Source: CAD feature listing. Evaluate the final solid. Frame: model axes, mm. Face numbers are marked on the shaded views. A direction names the side the tool comes from. Give positions to 0.01 mm unless a question says otherwise; leave off trailing zeros. Order: outer loops, then holes, each group sorted by start corner. A loop starts at its lowest first (then second) coordinate and runs counter-clockwise, first axis right, second up. Notation, with made-up numbers: M 78.5,-38.5 L 97.5,-38.5 A24 cw 97.5,-16.5 Z; hole C 33,-15 d11. An arc over 180 degrees is marked long. One line per question, with ' | ' between items. Start each with the question number.
from build123d import *

# Parameters (mm, degrees)
SKETCH_1_W               = 107
SKETCH_1_H               = 94
EXTRUDE_1_DEPTH          = 2
SKETCH_2_W               = 107
SKETCH_2_H               = 94
SKETCH_2_W_2             = 104
SKETCH_2_H_2             = 91
EXTRUDE_2_DEPTH          = 6.5
SKETCH_5_W               = 100
SKETCH_5_H               = 3.5
CUT_EXTRUDE_2_DEPTH      = 1.5
SKETCH_3_W               = 5
SKETCH_3_H               = 15
EXTRUDE_3_DEPTH          = 30
CUT_EXTRUDE_3_DEPTH      = 148.537283424
CUT_EXTRUDE_3_DEPTH_BACK = 30
SKETCH_6_W               = 3
SKETCH_6_H               = 9
SKETCH_7_W               = 10
SKETCH_7_H               = 15
EXTRUDE_4_DEPTH          = 2
SKETCH_8_R               = 1.5
CUT_EXTRUDE_4_DEPTH      = 2
CHAMFER_1_SIZE           = 0.5
EXTRUDE_5_DEPTH          = 3
EXTRUDE_6_DEPTH          = 3
EXTRUDE_7_DEPTH          = 3
MIRROR_2_COPY_1_DEPTH    = 3
EXTRUDE_8_DEPTH          = 15
EXTRUDE_9_DEPTH          = 15
EXTRUDE_10_DEPTH         = 9
EXTRUDE_11_DEPTH         = 9
EXTRUDE_12_DEPTH         = 3


with BuildPart() as part:
    # 草图1 → 凸台-拉伸1 (new body)
    with BuildSketch(Plane.XY):
        with Locations((53.5, -47)):
            Rectangle(SKETCH_1_W, SKETCH_1_H)
    extrude(amount=EXTRUDE_1_DEPTH)

    # 草图2 → 凸台-拉伸2 (add)
    with BuildSketch(Plane.XY.offset(2)):
        with Locations((53.5, -47)):
            Rectangle(SKETCH_2_W, SKETCH_2_H)
        with Locations((53.5, -47)):
            Rectangle(SKETCH_2_W_2, SKETCH_2_H_2, mode=Mode.SUBTRACT)
    extrude(amount=EXTRUDE_2_DEPTH)

    # 草图5 → 切除-拉伸2 (cut)
    with BuildSketch(Plane(origin=(0, -92.5, 0), x_dir=(1, 0, 0), z_dir=(0, 1, 0))):
        with Locations((53.5, -6.75)):
            Rectangle(SKETCH_5_W, SKETCH_5_H)
    extrude(amount=-CUT_EXTRUDE_2_DEPTH, mode=Mode.SUBTRACT)

    # 草图3 → 凸台-拉伸3 (add)
    with BuildSketch(Plane(origin=(0, 0, 0), x_dir=(-1, 0, 0), z_dir=(0, 0, -1))):
        with Locations((-2.5, -7.5)):
            Rectangle(SKETCH_3_W, SKETCH_3_H)
        with Locations((-104.5, -7.5)):
            Rectangle(SKETCH_3_W, SKETCH_3_H)
        with Locations((-2.5, -86.5)):
            Rectangle(SKETCH_3_W, SKETCH_3_H)
        with Locations((-104.5, -86.5)):
            Rectangle(SKETCH_3_W, SKETCH_3_H)
    extrude(amount=EXTRUDE_3_DEPTH)

    # 草图6 → 切除-拉伸3 (cut, two sides: drawn at the far end of the back side and taken through both)
    with BuildSketch(Plane(origin=(0, 0, -30), x_dir=(-1, 0, 0), z_dir=(0, 0, -1)).offset(-CUT_EXTRUDE_3_DEPTH_BACK)):
        with Locations((-103.5, -7.5)):
            Rectangle(SKETCH_6_W, SKETCH_6_H)
        with Locations((-103.5, -86.5)):
            Rectangle(SKETCH_6_W, SKETCH_6_H)
        with Locations((-3.5, -86.5)):
            Rectangle(SKETCH_6_W, SKETCH_6_H)
        with Locations((-3.5, -7.5)):
            Rectangle(SKETCH_6_W, SKETCH_6_H)
    extrude(amount=CUT_EXTRUDE_3_DEPTH + CUT_EXTRUDE_3_DEPTH_BACK, mode=Mode.SUBTRACT)

    # 草图7 → 凸台-拉伸4 (add)
    with BuildSketch(Plane(origin=(0, 0, -30), x_dir=(-1, 0, 0), z_dir=(0, 0, -1))):
        with Locations((5, -7.5)):
            Rectangle(SKETCH_7_W, SKETCH_7_H)
        with Locations((5, -86.5)):
            Rectangle(SKETCH_7_W, SKETCH_7_H)
        with Locations((-112, -7.5)):
            Rectangle(SKETCH_7_W, SKETCH_7_H)
        with Locations((-112, -86.5)):
            Rectangle(SKETCH_7_W, SKETCH_7_H)
    extrude(amount=-EXTRUDE_4_DEPTH)

    # 草图8 → 切除-拉伸4 (cut)
    with BuildSketch(Plane.XY.offset(-28)):
        with Locations((112.5, -7.5)):
            Circle(SKETCH_8_R)
        with Locations(Location((112.5, -86.5, 0), (0, 0, 180))):
            Circle(SKETCH_8_R)
        with Locations(Location((-5.5, -7.5, 0), (0, 0, 180))):
            Circle(SKETCH_8_R)
        with Locations((-5.5, -86.5)):
            Circle(SKETCH_8_R)
    extrude(amount=-CUT_EXTRUDE_4_DEPTH, mode=Mode.SUBTRACT)

    # 倒角1
    chamfer_1_edges = [part.edges().sort_by_distance(p)[0] for p in [
        (114, -86.5, -28),
        (-4, -7.5, -28),
        (-7, -86.5, -28),
        (111, -7.5, -28),
    ]]
    chamfer(chamfer_1_edges, length=CHAMFER_1_SIZE)

    # 草图9 → 凸台-拉伸5 (add)
    with BuildSketch(Plane.XZ.offset(94)):
        Polygon((87, 0), (102, -10), (102, 0), align=None)
        Polygon((5, 0), (20, 0), (5, -10), align=None)
    extrude_5 = extrude(amount=-EXTRUDE_5_DEPTH)

    # 草图10 → 凸台-拉伸6 (add)
    with BuildSketch(Plane(origin=(0, -79, 0), x_dir=(1, 0, 0), z_dir=(0, 1, 0))):
        Polygon((102, 10), (87, 0), (102, 0), align=None)
        Polygon((5, 0), (5, 10), (20, 0), align=None)
    extrude_6 = extrude(amount=-EXTRUDE_6_DEPTH)

    # 草图11 → 凸台-拉伸7 (add)
    with BuildSketch(Plane.ZY):
        Polygon((-20, -79), (0, -69), (0, -79), align=None)
    extrude_7 = extrude(amount=-EXTRUDE_7_DEPTH)

    # 镜向1: 凸台-拉伸7 across plane
    add(extrude_7.mirror(Plane(origin=(53.5, 0, 0), x_dir=(0, 0, 1), z_dir=(1, 0, 0))))

    # 镜向2: 凸台-拉伸5, 凸台-拉伸6, 凸台-拉伸7 across plane
    add(extrude_5.mirror(Plane.ZX.offset(-47)))
    add(extrude_6.mirror(Plane.ZX.offset(-47)))
    add(extrude_7.mirror(Plane.ZX.offset(-47)))

    # 镜向2 copy 1 sketch → 镜向2 copy 1 (add)
    with BuildSketch(Plane(origin=(107, -94, 0), x_dir=(0, 0, 1), z_dir=(1, 0, 0))):
        Polygon((-20, -79), (0, -69), (0, -79), align=None)
    extrude(amount=-MIRROR_2_COPY_1_DEPTH)

    # 草图12 → 凸台-拉伸8 (add)
    with BuildSketch(Plane(origin=(0, 0, 0), x_dir=(1, 0, 0), z_dir=(0, 1, 0))):
        Polygon((107, 25), (109, 28), (107, 28), align=None)
    extrude_8 = extrude(amount=-EXTRUDE_8_DEPTH)

    # 草图13 → 凸台-拉伸9 (add)
    with BuildSketch(Plane.XZ.offset(94)):
        Polygon((109, -28), (107, -25), (107, -28), align=None)
    extrude_9 = extrude(amount=-EXTRUDE_9_DEPTH)

    # 镜向3: 凸台-拉伸8, 凸台-拉伸9 across plane
    add(extrude_8.mirror(Plane(origin=(53.5, 0, 0), x_dir=(0, 0, 1), z_dir=(1, 0, 0))))
    add(extrude_9.mirror(Plane(origin=(53.5, 0, 0), x_dir=(0, 0, 1), z_dir=(1, 0, 0))))

    # 草图14 → 凸台-拉伸10 (add)
    with BuildSketch(Plane(origin=(0, -91, 0), x_dir=(1, 0, 0), z_dir=(0, 1, 0))):
        Polygon((2, 30), (2, 0), (20, 0), (5, 10), (5, 30), align=None)
        Polygon((102, 30), (102, 10), (87, 0), (105, 0), (105, 30), align=None)
    extrude(amount=EXTRUDE_10_DEPTH)

    # 草图15 → 凸台-拉伸11 (add)
    with BuildSketch(Plane.XZ.offset(3)):
        Polygon((105, -30), (105, 0), (87, 0), (102, -10), (102, -30), align=None)
        Polygon((5, -30), (5, -10), (20, 0), (2, 0), (2, -30), align=None)
    extrude(amount=EXTRUDE_11_DEPTH)

    # 草图17 → 凸台-拉伸12 (add)
    with BuildSketch(Plane.ZY):
        Polygon((-20, -15), (-20, -79), (0, -69), (0, -25), align=None)
    extrude_12 = extrude(amount=-EXTRUDE_12_DEPTH)

    # 镜向4: 凸台-拉伸12 across plane
    add(extrude_12.mirror(Plane(origin=(53.5, 0, 0), x_dir=(0, 0, 1), z_dir=(1, 0, 0))))


solid = part.part
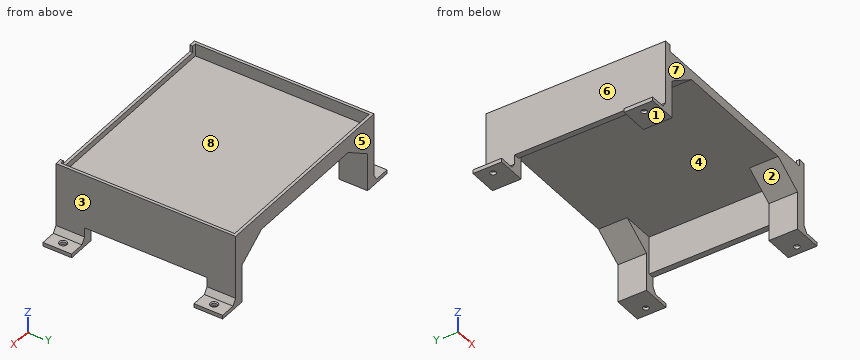
Item 1: Line query: line 1 (X direction, y = -86.5, z = -28.95); line 2 (Y direction, x = 112.5, z = -29.15); line 3 (X direction, y = -59.5, z = -7.5). Output: solid intervals per line, ascending.
Item 2: Cut plane C-C on x = 112.5. Return the cut outline in (y, z), and give its area (3 significant figures).
Item 3: Mould query, pull axis Y, two halves, no side actions, for the marked faces 6, 7 and 8. Classes: pulls with the +Y half, pulls with the -Y half, needs draft (parallel to the pull), parting line crosses it, or undercut.
Item 4: Pin query (flat end, axial travel): pin 1 Ø10 at (y, z) = (-28, -11) entering from -X; pin 2 Ø12 at (y, z) = (-10, -18) entering from +X; pin 3 Ø3 at (x, y) = (58, -82) entering from +Z. Return the tip coordinate at first contact, or that it passes through.
Item 5: Cut plane D-D on x = 21.5. Return the cut outline in (y, z).
Item 6: Reachability of the marked faces 1, 2, 3, 4 and 5 from +Z, -Z, +X, -X, +Y, -Y: full face, straight path, thin tool, end or side. Return the list, or none.
Item 7: Cut plane B-B on z = -5.5. Return the cut outline in (x, y).
Item 8: Cut plane A-A on y = -7.5. Count the separate pieces of the cut face and the enclosed holes in it, and give its area (3 significant figures).
Results are:
1) line 1: x = -10 to -7, -4 to 5, 102 to 111, 114 to 117 | line 2: y = -94 to -88, -85 to -79, -15 to -9, -6 to 0 | line 3: x = 0 to 3, 104 to 107
2) outline: M -94,-30 L -88,-30 L -88,-28.5 L -88.5,-28 L -94,-28 Z; M -85,-30 L -79,-30 L -79,-28 L -84.5,-28 L -85,-28.5 Z; M -15,-30 L -9,-30 L -9,-28.5 L -9.5,-28 L -15,-28 Z; M -6,-30 L 0,-30 L 0,-28 L -5.5,-28 L -6,-28.5 Z | area: 47.5 mm2
3) face 6: needs draft | face 7: pulls with the -Y half | face 8: undercut
4) pin 1: stops at x = 0 | pin 2: stops at x = 107 | pin 3: stops at z = 2
5) outline: M -94,0 L 0,0 L 0,8.5 L -1.5,8.5 L -1.5,2 L -92.5,2 L -92.5,5 L -94,5 Z
6) face 1: -Z, +X, -X, +Y, -Y | face 2: -Z, +Y, -Y | face 3: +Z, +X, +Y, -Y | face 4: -Z | face 5: +Z, -Z, +X, -X, +Y
7) outline: M 0,-94 L 11.75,-94 L 11.75,-79 L 3,-79 L 3,-15 L 11.75,-15 L 11.75,0 L 0,0 Z; M 95.25,-94 L 107,-94 L 107,0 L 95.25,0 L 95.25,-15 L 104,-15 L 104,-79 L 95.25,-79 Z
8) separate pieces: 3 | enclosed holes: 0 | area: 717 mm2
